Can you work these out from the model? Positions are in its coordinate system, mm. Give positions to 0.01 mm unless a question says otherwise; leave off trailing zeros. Order: outer loops, then holes, each group sorted by start corner. A loop starts at its lowest first (then second) coordinate and runs counter-clockwise, first axis right, second up. Notation, with made-up numbers: (6, 59) -> (34, 59) arc R34 cw to (34, 93) -> close; hole circle Ø10 at (71.25, 22). An arc over 180 degrees is marked (long way). Answer as a JSON object with one key per item and string values.
```python
from build123d import *

# Parameters (mm, degrees)
BOSS_EXTRUDE1_DEPTH   = 1.5875
F_1_0MM_DOWEL_HOLE1_D = 5.25
SKETCH6_R             = 3.45
CUT_EXTRUDE2_DEPTH    = 2.5
M4_CLEARANCE_HOLE1_D  = 4.5
M4_CLEARANCE_HOLE2_D  = 4.5
M4_CLEARANCE_HOLE3_D  = 4.5
M4_CLEARANCE_HOLE4_D  = 4.5


with BuildPart() as part:
    # Sketch1 → Boss-Extrude1 (new body, symmetric)
    with BuildSketch(Plane(origin=(0, 0, 0), x_dir=(1, 0, 0), z_dir=(0, 1, 0))):
        Polygon((-55, 15), (-30, 25), (30, 25), (55, 15), (55, -55), (-55, -55), align=None)
    extrude(amount=BOSS_EXTRUDE1_DEPTH, both=True)

    # Ø1.0mm Dowel Hole1 (through all)
    with Locations(Plane(origin=(0, 1.5875, 0), x_dir=(1, 0, 0), z_dir=(0, 1, 0))):
        with Locations((-20, 5), (20, 5), (45.980762114, -10), (-45.980762114, -10)):
            Hole(F_1_0MM_DOWEL_HOLE1_D / 2)

    # Sketch6 → Cut-Extrude2 (cut)
    with BuildSketch(Plane.XZ.offset(1.5875)):
        with Locations((-45.980762114, 10)):
            Circle(SKETCH6_R)
        with Locations((-20, -5)):
            Circle(SKETCH6_R)
        with Locations((20, -5)):
            Circle(SKETCH6_R)
        with Locations((45.980762114, 10)):
            Circle(SKETCH6_R)
    extrude(amount=-CUT_EXTRUDE2_DEPTH, mode=Mode.SUBTRACT)

    # M4 Clearance Hole1 (through all)
    with Locations(Plane(origin=(0, -1.5875, 0), x_dir=(-1, 0, 0), z_dir=(0, -1, 0))):
        with Locations((-24.440273443, -16.961605049), (-15.836626898, -29.248885713), (-44.91907455, -31.301015958), (-36.315428005, -43.588296622)):
            Hole(M4_CLEARANCE_HOLE1_D / 2)

    # M4 Clearance Hole2 (through all)
    with Locations(Plane(origin=(0, -1.5875, 0), x_dir=(-1, 0, 0), z_dir=(0, -1, 0))):
        with Locations((-5, 15), (5, 15)):
            Hole(M4_CLEARANCE_HOLE2_D / 2)

    # M4 Clearance Hole3 (through all)
    with Locations(Plane(origin=(0, 1.5875, 0), x_dir=(1, 0, 0), z_dir=(0, 1, 0))):
        with Locations((-15, -45), (15, -45)):
            Hole(M4_CLEARANCE_HOLE3_D / 2)

    # M4 Clearance Hole4 (through all)
    with Locations(Plane(origin=(0, 1.5875, 0), x_dir=(1, 0, 0), z_dir=(0, 1, 0))):
        with Locations((50, -20), (-50, -20)):
            Hole(M4_CLEARANCE_HOLE4_D / 2)


solid = part.part
```
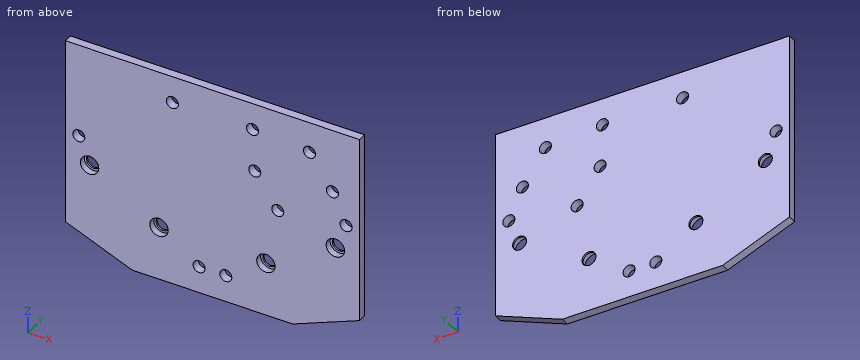
1. If we section it at B-B on z = 10: Please give me the cut outline in (x, y), then the cut area to 3 significant figures.
Worked answers:
{"outline": "(-55, -1.59) -> (-49.43, -1.59) -> (-49.43, 0.91) -> (-48.61, 0.91) -> (-48.61, 1.59) -> (-55, 1.59) -> close; (-43.36, 0.91) -> (-42.53, 0.91) -> (-42.53, -1.59) -> (42.53, -1.59) -> (42.53, 0.91) -> (43.36, 0.91) -> (43.36, 1.59) -> (-43.36, 1.59) -> close; (48.61, 0.91) -> (49.43, 0.91) -> (49.43, -1.59) -> (55, -1.59) -> (55, 1.59) -> (48.61, 1.59) -> close", "area": "308 mm²"}
2. Please list where these lines run through material, in increasing order: L1, parallel to X at y = 0.8, z = 20; L2, parallel to X at y = 1, z = 45; L3, parallel to Z at x = -20, y = 1.3 (3 decimals).
Worked answers:
{"L1": "-55 to -52.25, -47.75 to 47.75, 52.25 to 55", "L2": "-55 to -17.25, -12.75 to 12.75, 17.25 to 34.56, 38.07 to 55", "L3": "-25 to -7.625, -2.375 to 55"}
3. If we section it at D-D on z = -20: Please give me the cut outline in (x, y), then the cut area to 3 significant figures.
Worked answers:
{"outline": "(-42.5, -1.59) -> (42.5, -1.59) -> (42.5, 1.59) -> (-42.5, 1.59) -> close", "area": "270 mm²"}
4. Will these pins go through, and if not, where does the flat tip stop? pin 1 Ø2.5 at (x, z) = (15, 45) entering from +Y; pin 2 Ø6 at (x, z) = (45.98, 10) entering from -Y.
Worked answers:
{"pin 1": "through", "pin 2": "y = 0.91"}
5. If we section it at C-C on y = -0.75: Count the separate pieces of the cut face and the enclosed holes in it, then the cut area to 3 significant figures.
Worked answers:
{"separate pieces": "1", "enclosed holes": "14", "area": "8,240 mm²"}
